Here's the drawing with two shaded views (mm, measured from the low corner). I have some questions. Round coordinates to 2 decimals unless told otherwise and drop trailing zeros. Order: outer loops, then holes, each group sorted by start corner. A loop starts at its lowest first (then second) coordinate and runs counter-clockwise, first axis right, second up. Notation, with made-up numbers: (45.25, 85) -> (70.25, 85) arc R23 ccw to (70.25, 117) -> close; hole circle Ø4 at (49, 81). An arc over 180 degrees is marked (long way). Use a Markdown table: item, result. Add a question column.
Q1. We'd pull the mould along Z, two halves only. Please class the marked faces 1, 2, 3 and 4: +Z half, -Z half, draft (parallel to the pull), parting line (faces both ways), or undercut.
Q2. I need wall thicknesses on line 1 along Y through (x, z) = (54, 37.5) (1 decimal); line 2 along X through (y, z) = (85.5, 132) (1 decimal); line 3 along X through (y, z) = (18.5, 172.5) (1 decimal). Which ranges of each line are inside material? Lowest first, please. Write a range as [from, to].
Q3. I'm going to push flat-ended pins straight in: pin 1 Ø8 at (x, z) = (45.5, 57) entering from +Y; pin 2 Ø5 at (y, z) = (48, 119) entering from +X; pin 3 Ø1.5 at (x, y) = (67, 60) entering from +Z (1 decimal). Where does each tip first touch, or does it pass through?
Q4. If we section it at A-A on x = 47: List the corners of the cut face in (y, z) for me (1 decimal), plus the area to 3 significant figures.
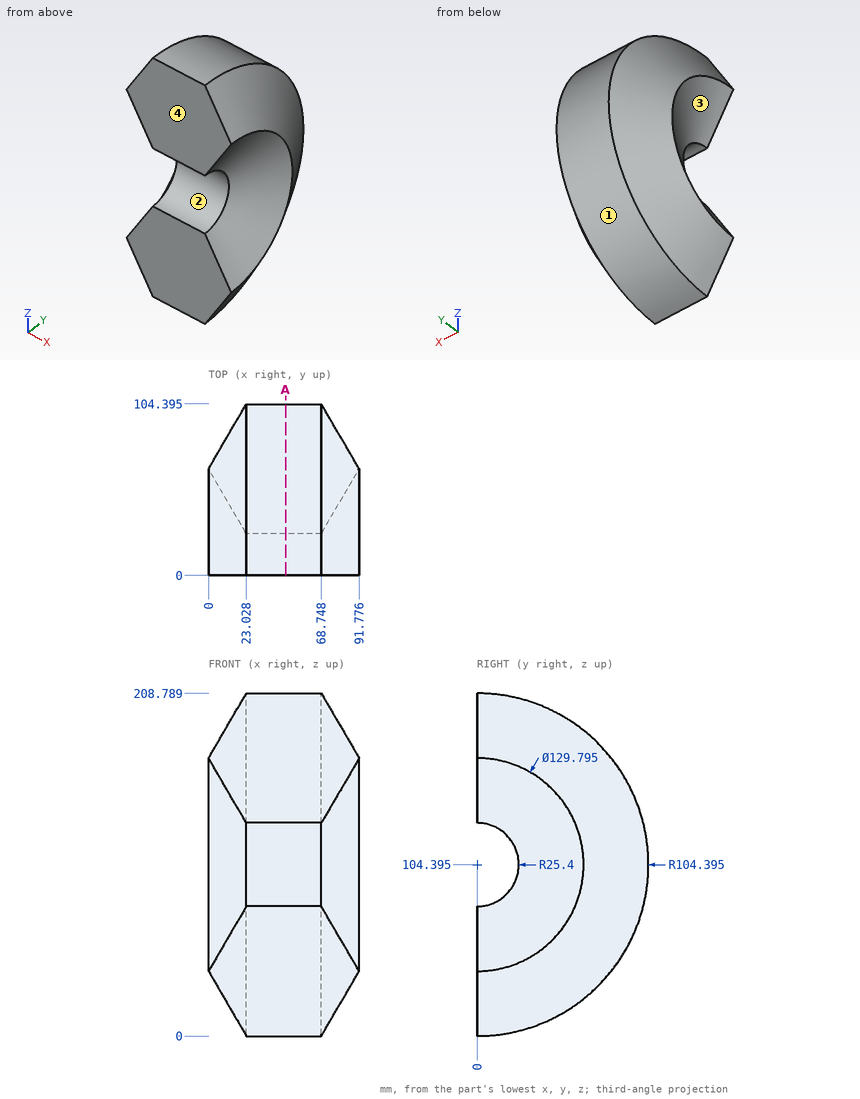
Answer below:
| question | item | result |
|---|---|---|
| 1 | face 1 | parting line |
| 1 | face 2 | undercut |
| 1 | face 3 | undercut |
| 1 | face 4 | draft |
| 2 | line 1 | [0, 80.1] |
| 2 | line 2 | [14.5, 77.2] |
| 2 | line 3 | [3.3, 88.5] |
| 3 | pin 1 | y = 94.95 |
| 3 | pin 2 | x = 84.65 |
| 3 | pin 3 | z = 190.3 |
| 4 | outline | (0, 0) arc R104.4 ccw to (0, 208.8) -> (0, 129.8) arc R25.4 cw to (0, 79) -> close |
| 4 | area | 16,100 mm² |
